from build123d import *

# Parameters (mm, degrees)
AUFSATZ_LINEAR_AUSTRAGEN1_DEPTH = 150
VERRUNDUNG1_R                   = 0.5
KREISMUSTER1_COUNT              = 4
SKIZZE3_W                       = 9
SKIZZE3_H                       = 9
AUFSATZ_LINEAR_AUSTRAGEN2_DEPTH = 150
SKIZZE4_R                       = 2.5
SCHNITT_LINEAR_AUSTRAGEN1_DEPTH = 151


with BuildPart() as part:
    # Skizze1 → Aufsatz-Linear austragen1 (new body)
    with BuildSketch(Plane.XY):
        Polygon((-0.707106781, 0.707106781), (6.585786438, 8), (3.1, 8), (3.1, 10), (10, 10), (10, 3.1), (8, 3.1), (8, 6.585786438), (0.707106781, -0.707106781), align=None)
    extrude(amount=AUFSATZ_LINEAR_AUSTRAGEN1_DEPTH)

    # Verrundung1
    verrundung1_edges = [part.edges().sort_by_distance(p)[0] for p in [
        (10, 3.1, 75),
        (8, 3.1, 75),
        (8, 6.585786438, 75),
        (6.585786438, 8, 75),
        (3.1, 8, 75),
        (3.1, 10, 75),
        (10, 10, 75),
    ]]
    fillet(verrundung1_edges, radius=VERRUNDUNG1_R)

    # Kreismuster1: part ×4 about axis
    kreismuster1_axis = Axis((0, 0, 0), (0, 0, 1))


with BuildPart() as part_1:
    add(part.part)
    for i in range(1, KREISMUSTER1_COUNT):
        add(part.part.rotate(kreismuster1_axis, i * 360 / KREISMUSTER1_COUNT))

    # Skizze3 → Aufsatz-Linear austragen2 (add)
    with BuildSketch(Plane.XY.offset(150)):
        Rectangle(SKIZZE3_W, SKIZZE3_H)
    extrude(amount=-AUFSATZ_LINEAR_AUSTRAGEN2_DEPTH)

    # Skizze4 → Schnitt-Linear austragen1 (cut, through all)
    with BuildSketch(Plane.XY.offset(150)):
        Circle(SKIZZE4_R)
    extrude(amount=-SCHNITT_LINEAR_AUSTRAGEN1_DEPTH, mode=Mode.SUBTRACT)


solid = part_1.part
For this review, take the finished solid that the model builds, in its own axes (mm). A direction names the side the tool comes from. Coordinates: 2 decimals unless noted, no trailing zeros. Order: outer loops, then holes, each group sorted by start corner. A loop starts at its lowest first (then second) coordinate and runs counter-clockwise, first axis right, second up. Notation, with made-up numbers: (33, 88.5) -> (87, 88.5) arc R23 ccw to (87, 124.5) -> close; hole circle Ø8 at (66, -31.5). An arc over 180 degrees is marked (long way). Return JSON: item names as keys, results as strings.
1. We need section A-A on y = 0. Write out the cut boundary in (x, z), and give its area (3 significant figures).
Answer block:
{"outline": "(-4.5, 0) -> (-2.5, 0) -> (-2.5, 150) -> (-4.5, 150) -> close; (2.5, 0) -> (4.5, 0) -> (4.5, 150) -> (2.5, 150) -> close", "area": "600 mm²"}
2. For line 1 (Y direction, x = 0, z = 56.5); line 2 (Y direction, x = -4, z = 59); line 3 (X direction, y = -5, z = 51), list the stretches that pass through material, from the lowest coordinate up. Write a range as from..to.
Answer block:
{"line 1": "-4.5..-2.5, 2.5..4.5", "line 2": "-10..-8, -5.41..5.41, 8..10", "line 3": "-10..-8, -6.41..-3.59, 3.59..6.41, 8..10"}
3. Machinability: for faces 1 (the flat face through (0, 4.5, 76)), 2 (the flat face through (-4.39, -5.805, 73.95)), 3 (the flat face through (0, -4.5, 76)), 4 (the flat face through (10, -7, 74)), 5 (the flat face through (4.5, 0, 76)), which of the approach directions +Z, -Z, +X, -X, +Y, -Y give a long, thin tool a straight path to every point of the face, cutting with its end or side? Answer none if there is none.
Answer block:
{"face 1": "+Z, -Z, +Y", "face 2": "+Z, -Z", "face 3": "+Z, -Z, -Y", "face 4": "+Z, -Z, +X, +Y, -Y", "face 5": "+Z, -Z, +X"}
4. For pin 1 Ø1.9 at (y, z) = (-1, 46.5) entering from +X, flat-tipped, find the tip position at first contact; note if it passes through.
Answer block:
{"pin 1": "x = 4.5"}
